```python
from build123d import *

# Parameters (mm, degrees)
SKETCH1_W               = 115
SKETCH1_H               = 140
BOSS_EXTRUDE1_DEPTH     = 6
CUT_EXTRUDE1_DEPTH      = 12
SKETCH5_R               = 2
CUT_EXTRUDE2_DEPTH      = 12
MIRROR2_COPY_1_DEPTH    = 12
MIRROR2_COPY_2_SKETCH_R = 2
MIRROR2_COPY_2_DEPTH    = 12


with BuildPart() as part:
    # Sketch1 → Boss-Extrude1 (new, symmetric)
    with BuildSketch(Plane.XY):
        Rectangle(SKETCH1_W, SKETCH1_H)
    extrude(amount=BOSS_EXTRUDE1_DEPTH, both=True)

    # Sketch4 → Cut-Extrude1 (cut)
    with BuildSketch(Plane.XY.offset(6)):
        with BuildLine():
            Line((52.5, 62), (52.5, 27))
            ThreePointArc((52.5, 27), (49.5, 24), (46.5, 27))
            Line((46.5, 27), (46.5, 62))
            ThreePointArc((46.5, 62), (49.5, 65), (52.5, 62))
        make_face()
    cut_extrude1 = extrude(amount=-CUT_EXTRUDE1_DEPTH, mode=Mode.SUBTRACT)

    # Sketch5 → Cut-Extrude2 (cut)
    with BuildSketch(Plane.XY.offset(6)):
        with Locations((37.5, 42)):
            Circle(SKETCH5_R)
    cut_extrude2 = extrude(amount=-CUT_EXTRUDE2_DEPTH, mode=Mode.SUBTRACT)

    # Mirror1: Cut-Extrude1, Cut-Extrude2 across plane
    add(cut_extrude1.mirror(Plane.ZX), mode=Mode.SUBTRACT)
    add(cut_extrude2.mirror(Plane.ZX), mode=Mode.SUBTRACT)

    # Mirror2: Cut-Extrude1, Cut-Extrude2 across plane
    add(cut_extrude1.mirror(Plane(origin=(0, 0, 0), x_dir=(0, 0, 1), z_dir=(1, 0, 0))), mode=Mode.SUBTRACT)
    add(cut_extrude2.mirror(Plane(origin=(0, 0, 0), x_dir=(0, 0, 1), z_dir=(1, 0, 0))), mode=Mode.SUBTRACT)

    # Mirror2 copy 1 sketch → Mirror2 copy 1 (cut)
    with BuildSketch(Plane(origin=(0, 0, 6), x_dir=(-1, 0, 0), z_dir=(0, 0, 1))):
        with BuildLine():
            Line((52.5, 62), (52.5, 27))
            ThreePointArc((52.5, 27), (49.5, 24), (46.5, 27))
            Line((46.5, 27), (46.5, 62))
            ThreePointArc((46.5, 62), (49.5, 65), (52.5, 62))
        make_face()
    extrude(amount=-MIRROR2_COPY_1_DEPTH, mode=Mode.SUBTRACT)

    # Mirror2 copy 2 sketch → Mirror2 copy 2 (cut)
    with BuildSketch(Plane(origin=(0, 0, 6), x_dir=(-1, 0, 0), z_dir=(0, 0, 1))):
        with Locations((37.5, 42)):
            Circle(MIRROR2_COPY_2_SKETCH_R)
    extrude(amount=-MIRROR2_COPY_2_DEPTH, mode=Mode.SUBTRACT)


solid = part.part
```
Input: part model. Units: mm. Frame: model coordinates. A direction names the side the tool comes from. Round coordinates to 2 decimals unless told otherwise and drop trailing zeros. Order: outer loops, then holes, each group sorted by start corner. A loop starts at its lowest first (then second) coordinate and runs counter-clockwise, first axis right, second up. Notation, with made-up numbers: (2, 27.5) - (61, 27.5) arc R13 ccw to (61, 47.5) - close; hole circle Ø8 at (87, 37.25). An arc over 180 degrees is marked (long way). One line per question, with ' | ' between items. Start each with the question number.
1) Cut plane A-A, the plane y = -42. Return the cut outline in (x, z), then the cut area to 3 significant figures.
2) Set-up query: faces 4 (the flat face through (-52.5, -45, 0)), 5 (the flat face through (-1, 1, 6)). Return all of +Z, -Z, +X, -X, +Y, -Y with unobstructed straight access to the full face (end or side cutting, diameter ignored); none if empty.
3) Contact query for a flat-ended pin moving along its axis: P1, Ø3.5, axis at x = -37.5, y = 42, coming from the +Z side. Output: stop coordinate, or through.
4) Cut plane D-D, the plane x = -49.5. Return the cut outline in (y, z), then the cut area to 3 significant figures.
5) Cut plane B-B, the plane x = 37.5. Return the cut outline in (y, z).
6) Cut plane C-C, the plane z = -0.75. Give the number of separate pieces and of enclosed holes in the cut face, then the cut area to 3 significant figures.
7) Ray query, probe 1 along X at (y, z) = (57, -1.5); probe 2 along X at (y, z) = (-42, -0.75); probe 3 along Y at (x, z) = (-37.5, -1). Return the intervals inside material, ascending.
8) Pull-direction query (Y, two-part tool) for faces 1 (the flat face through (-46.5, 44, 0)), 2 (the flat face through (-1, 70, 0)), 3 (the flat face through (-57.5, -1, 0)); classes: +Y half, -Y half, draft (parallel to the pull), parting line (faces both ways), or undercut.
Worked out:
1) outline: (-57.5, -6) - (-52.5, -6) - (-52.5, 6) - (-57.5, 6) - close; (-46.5, -6) - (-39.5, -6) - (-39.5, 6) - (-46.5, 6) - close; (-35.5, -6) - (35.5, -6) - (35.5, 6) - (-35.5, 6) - close; (39.5, -6) - (46.5, -6) - (46.5, 6) - (39.5, 6) - close; (52.5, -6) - (57.5, -6) - (57.5, 6) - (52.5, 6) - close | area: 1,140 mm^2
2) face 4: +Z, -Z | face 5: +Z, +X, -X, +Y, -Y
3) P1: passes through
4) outline: (-70, -6) - (-65, -6) - (-65, 6) - (-70, 6) - close; (-24, -6) - (24, -6) - (24, 6) - (-24, 6) - close; (65, -6) - (70, -6) - (70, 6) - (65, 6) - close | area: 696 mm^2
5) outline: (-70, -6) - (-44, -6) - (-44, 6) - (-70, 6) - close; (-40, -6) - (40, -6) - (40, 6) - (-40, 6) - close; (44, -6) - (70, -6) - (70, 6) - (44, 6) - close
6) separate pieces: 1 | enclosed holes: 8 | area: 15,100 mm^2
7) probe 1: x = -57.5 to -52.5, -46.5 to 46.5, 52.5 to 57.5 | probe 2: x = -57.5 to -52.5, -46.5 to -39.5, -35.5 to 35.5, 39.5 to 46.5, 52.5 to 57.5 | probe 3: y = -70 to -44, -40 to 40, 44 to 70
8) face 1: undercut | face 2: +Y half | face 3: draft
